```python
from build123d import *

# Parameters (mm, degrees)
BOSS_EXTRUDE1_DEPTH = 30
SKETCH2_R           = 3
CUT_EXTRUDE1_DEPTH  = 111
SKETCH3_R           = 3
CUT_EXTRUDE2_DEPTH  = 111
FILLET1_R           = 5
FILLET2_R           = 5
FILLET3_R           = 15


with BuildPart() as part:
    # Sketch1 → Boss-Extrude1 (new body)
    with BuildSketch(Plane.XY):
        Polygon((0, 0), (51, 0), (51, -100), (41, -100), (41, -73), (10, -73), (10, -100), (0, -100), align=None)
    extrude(amount=BOSS_EXTRUDE1_DEPTH)

    # Sketch2 → Cut-Extrude1 (cut)
    with BuildSketch(Plane(origin=(51, 0, 0), x_dir=(0, 0, -1), z_dir=(1, 0, 0))):
        with Locations(Location((-15, -85, 0), (0, 0, 90))):
            Circle(SKETCH2_R)
    extrude(amount=-CUT_EXTRUDE1_DEPTH, mode=Mode.SUBTRACT)

    # Sketch3 → Cut-Extrude2 (cut)
    with BuildSketch(Plane(origin=(0, 0, 0), x_dir=(-1, 0, 0), z_dir=(0, 0, -1))):
        with Locations((-25.5, -15)):
            Circle(SKETCH3_R)
        with Locations((-25.5, -30)):
            Circle(SKETCH3_R)
        with Locations((-25.5, -50)):
            Circle(SKETCH3_R)
    extrude(amount=-CUT_EXTRUDE2_DEPTH, mode=Mode.SUBTRACT)

    # Fillet1
    fillet1_edges = [part.edges().sort_by_distance(p)[0] for p in [
        (0, -50, 0),
        (25.5, 0, 0),
        (51, -50, 0),
    ]]
    fillet(fillet1_edges, radius=FILLET1_R)

    # Fillet2
    fillet2_edges = [part.edges().sort_by_distance(p)[0] for p in [
        (51, -50, 30),
        (0, -50, 30),
    ]]
    fillet(fillet2_edges, radius=FILLET2_R)

    # Fillet3
    fillet3_edges = [part.edges().sort_by_distance(p)[0] for p in [
        (25.5, -73, 30),
        (25.5, -73, 0),
    ]]
    fillet(fillet3_edges, radius=FILLET3_R - 0.0001)  # a hair under: the kernel refuses the full size


solid = part.part
```
Source: CAD feature listing. Evaluate the final solid. Frame: model axes, mm. A direction names the side the tool comes from. Coordinates: 2 decimals unless noted, no trailing zeros. Loops run counter-clockwise (first coordinate to the right, second up) from the corner with the lowest first, then second, coordinate; pieces in that order, holes last. Notation, with made-up numbers: M 0,10 L 7,10 A16 ccw 7,31 Z; hole C 58.25,-27 d1. An arc over 180 degrees is marked long. Use a Markdown table: item, result. Add a question column.
Q1. Section query C-C, the plane y = -85. Return loops of the section in (x, z), and give its area (3 significant figures).
Q2. Access query for faces 1 (the cylindrical face through (25.28, -68.49, 4.28)), 2 (the cylindrical face through (46.1, -87.4, 13.2)). Directions: +Z, -Z, +X, -X, +Y, -Y. A direction counts if a zero-diameter tool reaches every point of the face in a straight line with its end or side. Return the directions, or none.
Q3. Section query B-B, the plane z = 13.5. Return loops of the section in (x, y), and give its area (3 significant figures).
Q4. Material intervals for L1, parallel to Y at x = 25.5, z = 12; L2, parallel to Z at x = 5, y = -85; L3, parallel to Y at x = 25.5, z = 9, sorted ascending.
Q5. Draft query along X for faces 3 (the flat face through (5, -100, 15)), 4 (the cylindrical face through (1, -49, 28)), 5 (the cylindrical face through (25.28, -68.49, 25.72)), 6 (the cylindrical face through (25.891, -47.026, 14.79)). Return one class per face: pulls with the +X half, pulls with the -X half, needs draft (parallel to the pull), parting line crosses it, or undercut.
Q6. Section query A-A, the plane y = -15. Return loops of the section in (x, z), and give its area (3 significant figures).
Q7. First-contact query: pin 1 (3.5 mm diameter, centred on y = -85, z = 15, fed in from -X); pin 2 (10 mm diameter, centred on x = 26, z = 14, fed in from -Y). Flat tips, straight axial feed; report the tip coordinate or a pass-through.
Result:
| question | item | result |
|---|---|---|
| 1 | outline | M 0,5 A5 ccw 5,0 L 10,0 L 10,12 L 0,12 Z; M 0,18 L 10,18 L 10,30 L 5,30 A5 ccw 0,25 Z; M 41,0 L 46,0 A5 ccw 51,5 L 51,12 L 41,12 Z; M 41,18 L 51,18 L 51,25 A5 ccw 46,30 L 41,30 Z |
| 1 | area | 459 mm2 |
| 2 | face 1 | -Z, -Y |
| 2 | face 2 | +X, -X |
| 3 | outline | M 0,-100 L 10,-100 L 10,-87.6 L 0,-87.6 Z; M 0,-82.4 L 10,-82.4 L 10,-72.92 L 41,-72.92 L 41,-82.4 L 51,-82.4 L 51,0 L 0,0 Z; M 41,-100 L 51,-100 L 51,-87.6 L 41,-87.6 Z; hole C 25.5,-50 d6; hole C 25.5,-30 d6; hole C 25.5,-15 d6 |
| 3 | area | 4,070 mm2 |
| 4 | L1 | y = -72.7 to -53, -47 to -33, -27 to -18, -12 to 0 |
| 4 | L2 | z = 0 to 12, 18 to 30 |
| 4 | L3 | y = -71.75 to -53, -47 to -33, -27 to -18, -12 to 0 |
| 5 | face 3 | needs draft |
| 5 | face 4 | pulls with the -X half |
| 5 | face 5 | undercut |
| 5 | face 6 | undercut |
| 6 | outline | M 0,5 A5 ccw 5,0 L 22.5,0 L 22.5,30 L 5,30 A5 ccw 0,25 Z; M 28.5,0 L 46,0 A5 ccw 51,5 L 51,25 A5 ccw 46,30 L 28.5,30 Z |
| 6 | area | 1,330 mm2 |
| 7 | pin 1 | passes through |
| 7 | pin 2 | stops at y = -73 |
